```python
from build123d import *

# Parameters (mm, degrees)
SKETCH001_W           = 11.5
SKETCH001_H           = 4
SKETCH002_W           = 23
SKETCH002_H           = 23
POCKET_DEPTH          = 2
FILLET_R              = 3
SKETCH008_R           = 1.6
POCKET004_DEPTH       = 123.064009
POLARPATTERN001_COUNT = 3


with BuildPart() as part:
    # Sketch001 → Revolution001 (revolve)
    with BuildSketch(Plane.XZ):
        with Locations((-15.25, -2)):
            Rectangle(SKETCH001_W, SKETCH001_H)
    revolve(axis=Axis((0, 0, 0), (0, 0, 1)))

    # Sketch002 (on Face3 of Revolution001) → Pocket (cut)
    with BuildSketch(Plane(origin=(0, 0, -4), x_dir=(1, 0, 0), z_dir=(0, 0, -1))):
        Rectangle(SKETCH002_W, SKETCH002_H)
    extrude(amount=-POCKET_DEPTH, mode=Mode.SUBTRACT)

    # Fillet
    fillet_edges = [part.edges().sort_by_distance(p)[0] for p in [
        (-11.5, 11.5, -3),
        (11.5, 11.5, -3),
        (11.5, -11.5, -3),
        (-11.5, -11.5, -3),
    ]]
    fillet(fillet_edges, radius=FILLET_R)

    # Sketch008 → Pocket004 (cut, through all)
    with BuildSketch(Plane(origin=(0, 0, -4), x_dir=(1, 0, 0), z_dir=(0, 0, -1))):
        with Locations((17.8, 0)):
            Circle(SKETCH008_R)
    pocket004 = extrude(amount=-POCKET004_DEPTH, mode=Mode.SUBTRACT)

    # PolarPattern001: Pocket004 ×3 about axis
    polarpattern001_axis = Axis((0, 0, -4), (0, 0, -1))
    for i in range(1, POLARPATTERN001_COUNT):
        add(pocket004.rotate(polarpattern001_axis, i * 360 / POLARPATTERN001_COUNT), mode=Mode.SUBTRACT)


solid = part.part
```
Read the model definition and answer for the solid it produces. Units are mm, in the model's axes. A direction names the side the tool comes from. Coordinates: 2 decimals unless noted, no trailing zeros. Loops run counter-clockwise (first coordinate to the right, second up) from the corner with the lowest first, then second, coordinate; pieces in that order, holes last.
(1) Flat-ended cylindrical pins translate along their axes: pin 1 Ø0.6 at (y, z) = (3, -3) entering from -X; pin 2 Ø1.6 at (x, z) = (0.5, -3) entering from -Y; pin 3 Ø1 at (x, z) = (-9, -1.5) entering from -Y. Find the tip coordinate at first contact, or state that the pin passes through.
Solution:
pin 1: stops at x = -20.83
pin 2: stops at y = -21
pin 3: stops at y = -19.2
(2) The mould has two halves that part along X. Classify faces 1 (the face through (-20.03, -6.31, -1.97)), 2 (the face through (0, -11.5, -3)), 3 (the face through (-4, 9, 0)): released by +X, released by -X, zero draft, split by the parting line, or undercut.
Solution:
face 1: split by the parting line
face 2: undercut
face 3: zero draft
(3) Consider line 1 along X through (y, z) = (0, -1.4); line 2 along X through (y, z) = (0, -2.7); line 3 along Y through (x, z) = (0, -2.35). Determine where each line is inside the solid, lowest interval first.
Solution:
line 1: x = -21 to -9.5, 9.5 to 16.2, 19.4 to 21
line 2: x = -21 to -11.5, 11.5 to 16.2, 19.4 to 21
line 3: y = -21 to -11.5, 11.5 to 21
(4) The part is cut by section D-D (y = 16). Determine the outline of the cut face in (x, z).
Solution:
outline: (-13.6, -4) - (-10.39, -4) - (-10.39, 0) - (-13.6, 0) - close; (-7.41, -4) - (13.6, -4) - (13.6, 0) - (-7.41, 0) - close
(5) The part is cut by section A-A (y = 0). Determine the outline of the cut face in (x, z), and give its area (3 significant figures).
Solution:
outline: (-21, -4) - (-11.5, -4) - (-11.5, -2) - (-9.5, -2) - (-9.5, 0) - (-21, 0) - close; (9.5, -2) - (11.5, -2) - (11.5, -4) - (16.2, -4) - (16.2, 0) - (9.5, 0) - close; (19.4, -4) - (21, -4) - (21, 0) - (19.4, 0) - close
area: 71.2 mm2
(6) A tool of negligible diameter and unlimited length cuts with its end or side. For faces 4 (the face through (10.6, -10.64, -2.99)), 5 (the face through (-9.11, -17, -2.03)), from which of +Z, -Z, +X, -X, +Y, -Y can it reach the whole face along a straight path? Write none if from no direction.
Solution:
face 4: -Z
face 5: +Z, -Z
(7) The part is cut by section C-C (z = -3.5). Determine the outline of the cut face in (x, y), and give its area (3 significant figures).
Solution:
outline: circle Ø42 at (0, 0); hole (-11.5, -8.5) arc R3 ccw to (-8.5, -11.5) - (8.5, -11.5) arc R3 ccw to (11.5, -8.5) - (11.5, 8.5) arc R3 ccw to (8.5, 11.5) - (-8.5, 11.5) arc R3 ccw to (-11.5, 8.5) - close; hole circle Ø3.2 at (-8.9, -15.42); hole circle Ø3.2 at (-8.9, 15.42); hole circle Ø3.2 at (17.8, 0)
area: 840 mm2
(8) The part is cut by section B-B (x = 0). Determine the outline of the cut face in (y, z).
Solution:
outline: (-21, -4) - (-11.5, -4) - (-11.5, -2) - (-9.5, -2) - (-9.5, 0) - (-21, 0) - close; (9.5, -2) - (11.5, -2) - (11.5, -4) - (21, -4) - (21, 0) - (9.5, 0) - close
